Build history of the part. All positions in model axes, mm. A direction names the side the tool comes from. Coordinates: 2 decimals unless noted, no trailing zeros. Loops run counter-clockwise (first coordinate to the right, second up) from the corner with the lowest first, then second, coordinate; pieces in that order, holes last.
(1) Slice it at C-C (z = -72). Give the cut face in (x, y).
(2) Flat gauge pins, fed straight in: P1, Ø0.8, axis at x = -8, y = 1, coming from the -Z side; P2, Ø0.5, axis at x = -8.5, y = 0.5, coming from the +Z side; P3, Ø4, axis at x = -33.1, z = -49.15, coming from the -Y side; P4, Ø0.5, axis at x = -8.5, y = 1, coming from the -Z side. Where does each tip first touch, or does it go through?
(3) Wall check: L1, parallel to Z at x = -34, y = 0.7; L2, parallel to Z at x = -17, y = 0.8; L3, parallel to X at y = 0.9, z = -42.5. Give the ranges that are in metal, low to high.
(4) Two-plate mould, pull along X, no slides. Class faces 3 (the face through (-36.171, 0.783, -115.884)), 4 (the face through (-32.183, 0.805, -102.146)), 5 (the face through (-1.003, 0.783, -18.351)): pulls with the +X half, pulls with the -X half, needs draft (parallel to the pull), parting line crosses it, or undercut.
(5) Slice it at D-D (x = -37). Give the cut face in (y, z).
(6) Slice it at B-B (y = 0.7). Give the number of separate pieces and of enclosed holes in the cut face, and give its area (3 significant figures).
(7) Slice it at A-A (x = -14). Give the cut face in (y, z), and give its area (3 significant figures).
(8) Tool access for faces 1 (the face through (-43.055, 0.783, -48.29)), 2 (the face through (-4.07, 0.8, -36.39)): list every direction of +Z, -Z, +X, -X, +Y, -Y with a clear straight run to the whole face (end or side of a thin tool).
Autodesk Inventor part; units mm, degrees
ref_plane "YZ Plane" through (0, 0, 0) normal (1, 0, 0) x (0, 1, 0)
ref_plane "XZ Plane" through (0, 0, 0) normal (0, 1, 0) x (-1, 0, 0)
ref_plane "XY Plane" through (0, 0, 0) normal (0, 0, 1) x (1, 0, 0)
sketch "Sketch2" plane through (0, 0, 0) normal (0, 1, 0) x (-1, 0, 0)
  line L0 (50.8978, -88.9331) -> (25.3484, -88.9331)
  line L1 (25.3484, -88.9331) -> (25.3484, -76.2331)
  line L2 (25.3484, -76.2331) -> (0.0063, -76.2331)
  line L3 (50.8978, -88.9331) -> (50.8978, -113.4067)
  line L4 (0.0063, -76.2331) -> (0.0055, -63.5331)
  line L5 (0.0055, -63.5331) -> (-22.2195, -63.5346)
  arc A0 (-20.3669, -62.9196) -> (-2.754, -47.4243) centre (-31.4849, -32.5245) ccw
  arc A1 (48.1058, -116.5585) -> (50.8978, -113.4067) centre (47.7228, -113.4067) ccw
  arc A2 (-20.3669, -62.9196) -> (-20.967, -65.5097) centre (-19.8216, -64.4105) ccw
  arc A3 (-2.754, -47.4243) -> (0.0978, -35.7707) centre (-25.3022, -35.7309) ccw
  line L6 (0.0978, -4.698) -> (47.7219, -4.6852)
  line L7 (50.8978, -7.8602) -> (50.8978, -88.9331)
  line L8 (0.0978, -20.5717) -> (0.0978, -35.7707)
  line L9 (3.2719, -4.6971) -> (12.7978, -4.6946)
  line L10 (12.7978, -4.6946) -> (12.8012, -17.3967)
  line L11 (12.8012, -17.3967) -> (20.9, -17.3945)
  line L12 (38.2012, -17.3899) -> (38.2012, -93.5899)
  line L13 (12.8012, -17.3967) -> (12.8012, -68.1967)
  arc A4 (50.8978, -7.8602) -> (47.7219, -4.6852) centre (47.7228, -7.8602) ccw
  arc A5 (3.2719, -4.6971) -> (0.0978, -7.8721) centre (3.2728, -7.8721) ccw
  line L14 (12.8012, -68.1967) -> (12.8012, -74.5467)
  line L15 (38.2012, -93.5899) -> (38.2012, -99.9399)
  line L16 (38.2012, -17.3899) -> (38.2012, -23.7399)
  line L17 (12.8012, -17.3967) -> (12.8012, -23.7467)
  line L18 (12.8012, -23.7467) -> (19.1512, -23.7467)
  line L19 (19.1512, -23.7467) -> (6.4512, -23.7467)
  line L20 (25.3484, -88.9331) -> (31.6984, -88.9331)
  line L21 (31.6984, -88.9331) -> (31.6984, -114.3331)
  arc A6 (-20.967, -65.5097) -> (31.6984, -114.3331) centre (249.7999, 173.7477) ccw
  arc A7 (31.6984, -114.3331) -> (33.1489, -115.4256) centre (249.7999, 173.7477) ccw
  line L22 (38.2012, -88.9331) -> (38.2012, -69.8831)
  line L23 (38.2012, -69.8831) -> (44.7036, -69.8831)
  line L24 (38.2012, -17.3899) -> (16.8506, -17.3956)
  line L25 (12.8012, -17.3967) -> (3.2728, -17.3967)
  arc A8 (38.2012, -113.7028) -> (38.2012, -17.3899) centre (-135.4238, -65.5464) ccw
  arc A9 (33.1489, -115.4256) -> (38.2012, -113.7028) centre (35.0868, -112.839) ccw
  arc A10 (3.2728, -17.3967) -> (0.0978, -20.5717) centre (3.2728, -20.5717) ccw
  line L26 (38.2012, -17.3899) -> (16.8506, -17.3956)
  arc A11 (44.7558, -65.5464) -> (30.4886, -17.392) centre (-43.6427, -65.5464) ccw
  arc A12 (38.2012, -32.1417) -> (24.6857, -17.3935) centre (11.5084, -43.0364) ccw
  arc A13 (32.7636, -23.5578) -> (27.4631, -19.2197) centre (15.0605, -39.7812) ccw
  arc A14 (27.4631, -19.2197) -> (20.9, -17.3945) centre (20.9035, -30.0945) ccw
  line L27 (0.0978, -20.5717) -> (31.8478, -20.5717)
  line L28 (31.8478, -20.5717) -> (31.8478, -76.2331)
  line L29 (31.8478, -17.3916) -> (31.8478, -74.5467)
  line L30 (31.8478, -74.5467) -> (31.6984, -99.9463)
  line L31 (31.6984, -99.9463) -> (31.5861, -119.0417)
  line L32 (31.6984, -99.9463) -> (31.6984, -49.1463)
  line L33 (31.6984, -99.9463) -> (82.4984, -99.9463) construction
  line L34 (31.6984, -49.1463) -> (33.0954, -49.1463)
  line L35 (31.6984, -99.9463) -> (33.0954, -99.9463)
  point P0 (0, 0)
  point P1 (50.8978, -120.6831)
  point P2 (0.0775, -39.6857)
  point P3 (-21.1455, -63.5345)
  point P4 (50.8978, -4.6844)
  point P5 (3.2719, -4.6971)
  point P6 (38.0838, -119.0579)
  point P7 (23.7439, -17.3938)
  point P8 (12.8012, -17.3967)
  dimension "d3" = 12.7
  dimension "d4" = 31.75
  dimension "d5" = 12.7
  dimension "d6" = 22.225
  dimension "d18" = 3.175
  dimension "d19" = 1.5875
  dimension "d23" = 4.699
  dimension "d24" = 12.7
  dimension "d25" = 25.4
  dimension "d26" = 76.2
  dimension "d27" = 50.8
  dimension "d28" = 3.175
  dimension "d33" = 6.35
  dimension "d35" = 6.35
  dimension "d36" = 6.35
  dimension "d37" = 6.35
  dimension "d38" = 12.7
  dimension "d54" = 6.35
  dimension "d55" = 25.4
  dimension "d56" = 50.8
  dimension "d58" = 19.05
  dimension "d59" = 3.175
  dimension "d60" = 12.7
  dimension "d61" = 31.75
  dimension "d62" = 25.4
  dimension "d63" = 19.0957
  dimension "d64" = 180
  dimension "d65" = 50.8
  dimension "d66" = 90
  dimension "d69" = 1.397
extrude "Extrusion1" add sketch "Sketch2" along normal blind 1.5875 contours L21 L31 A6 A2 L5 L4 L2 L1 L0 | L32 L34 L28 L30 L0 | L0 L30 L21 | L0 L1 L2 L4 L5 A2 A0 A3 L8 L27 A13 L28 L34 L32 | L30 L28 A12 L12 L0 | L0 A8 A9 A7 L21 L30 | L21 A6 L31 | L12 L23 A8 L0 | L12 A11 A8 L23 | L27 L13 L11 A14 A13 | L27 A10 L25 L13
hole "Hole3" at (-6.4512, 0, -23.7467) at (-19.1512, 0, -23.7467) at (-12.8012, 0, -68.1967) at (-33.0954, 0, -49.1463) at (-33.0954, 0, -99.9463) direction (0, 1, 0) diameter 4.7625 end through all
sketch "Sketch3" plane through (0, 1.5875, 0) normal (0, 1, 0) x (1, 0, 0)
  circle A0 centre (-19.1512, 23.7467) radius 2.3813
  line L0 (-19.1512, 23.7467) -> (-19.1512, 42.7967) construction
  line L1 (-19.1512, 23.7467) -> (-0.1012, 23.7467) construction
  line L2 (-19.1512, 42.7967) -> (-12.8012, 42.7967)
  circle A1 centre (-6.4512, 23.7467) radius 2.3813
  line L3 (-6.4512, 23.7467) -> (-6.4512, 36.4467) construction
  line L4 (-6.4512, 36.4467) -> (-19.1512, 36.4467) construction
  arc A2 (-19.1512, 38.828) -> (-19.1512, 34.0655) centre (-19.1512, 36.4467) ccw
  arc A3 (-6.4512, 34.0655) -> (-6.4512, 38.828) centre (-6.4512, 36.4467) ccw
  line L5 (-19.1512, 34.0655) -> (-6.4512, 34.0655)
  line L6 (-6.4512, 36.4467) -> (-6.4512, 49.1467) construction
  line L7 (-6.4512, 49.1467) -> (-19.1512, 49.1467) construction
  arc A4 (-19.1512, 51.528) -> (-19.1512, 46.7655) centre (-19.1512, 49.1467) ccw
  arc A5 (-6.4512, 46.7655) -> (-6.4512, 51.528) centre (-6.4512, 49.1467) ccw
  line L8 (-6.4512, 51.528) -> (-19.1512, 51.528)
  line L9 (-12.8012, 34.0655) -> (-12.8012, 36.4467)
  line L10 (-12.8012, 36.4467) -> (-19.1512, 36.4467)
  line L11 (-19.1512, 38.828) -> (-15.9722, 38.828)
  line L12 (-6.4512, 38.828) -> (-9.6302, 38.828)
  line L13 (-6.4512, 46.7655) -> (-9.1999, 46.7655)
  line L14 (-19.1512, 46.7655) -> (-16.4024, 46.7655)
  arc A6 (-9.7971, 39.2979) -> (-9.3895, 46.3163) centre (-12.8012, 42.9934) ccw
  arc A7 (-16.2129, 46.3163) -> (-15.8053, 39.2979) centre (-12.8012, 42.9934) ccw
  arc A8 (-9.7971, 39.2979) -> (-9.6302, 38.828) centre (-9.6302, 39.0926) ccw
  arc A9 (-15.9722, 38.828) -> (-15.8053, 39.2979) centre (-15.9722, 39.0926) ccw
  arc A10 (-16.2129, 46.3163) -> (-16.4024, 46.7655) centre (-16.4024, 46.5009) ccw
  arc A11 (-9.1999, 46.7655) -> (-9.3895, 46.3163) centre (-9.1999, 46.5009) ccw
  point P0 (0, 0)
  point P1 (-15.1101, 38.828)
  point P2 (-10.4923, 38.828)
  point P3 (-9.8938, 46.7655)
  point P4 (-15.7085, 46.7655)
  dimension "d70" = 19.05
  dimension "d71" = 90
  dimension "d72" = 6.35
  dimension "d73" = 12.7
  dimension "d78" = 6.35
  dimension "d79" = 0.2646
extrude "Extrusion2" cut sketch "Sketch3" against normal through all contours L11 A9 A7 A10 L14 A4 L8 A5 L13 A11 A6 A8 L12 A3 L5 A2
properties part number "sled2" material "Polycarbonate, Smoke"
Response values:
1. outline: (-44.64, 0) - (15.09, 0) - (15.09, 1.59) - (-44.64, 1.59) - close
2. P1: stops at z = -95.11
2. P2: stops at z = -17.4
2. P3: passes through
2. P4: stops at z = -95.42
3. L1: z = -115.88 to -102.15, -97.74 to -51.35, -46.94 to -25
3. L2: z = -102.59 to -51.53, -46.77 to -45.24, -40.75 to -38.83, -34.07 to -24.77, -22.73 to -17.4
3. L3: x = -41.7 to -17.54, -8.06 to 0.82
4. face 3: parting line crosses it
4. face 4: undercut
4. face 5: pulls with the +X half
5. outline: (0, -115.44) - (1.59, -115.44) - (1.59, -29.57) - (0, -29.57) - close
6. separate pieces: 1
6. enclosed holes: 6
6. area: 3,710 mm2
7. outline: (0, -100.04) - (1.59, -100.04) - (1.59, -70.25) - (0, -70.25) - close; (0, -66.14) - (1.59, -66.14) - (1.59, -51.53) - (0, -51.53) - close; (0, -34.07) - (1.59, -34.07) - (1.59, -17.4) - (0, -17.4) - close
7. area: 96.9 mm2
8. face 1: +Z, -X, +Y, -Y
8. face 2: +Y, -Y
